Can you work these out from the model? Positions are in its coordinate system, mm. Face numbers are marked on the shaded views. Give positions to 0.01 mm unless a question says otherwise; leave off trailing zeros. Order: outer loops, then holes, each group sorted by start corner. A loop starts at its lowest first (then second) coordinate and runs counter-clockwise, first axis right, second up. Notation, with made-up numbers: (82.25, 23) -> (132.25, 23) arc R20 cw to (132.25, 29) -> close; hole circle Ø2 at (7.5, 86). An arc over 180 degrees is marked (long way). Answer as CSV lines item,"result".
```python
from build123d import *

# Parameters (mm, degrees)
EXTRUDE_1_DEPTH     = 20
SKETCH_2_R          = 1.5
CUT_EXTRUDE_1_DEPTH = 2.5


with BuildPart() as part:
    # 草图1 → 凸台-拉伸1 (new, symmetric)
    with BuildSketch(Plane.XY):
        Polygon((-4.5, 4.5), (4.5, 4.5), (4.5, 0), (13.5, 0), (13.5, 8), (-13.5, 8), (-13.5, 0), (-4.5, 0), align=None)
    extrude(amount=EXTRUDE_1_DEPTH, both=True)

    # 草图2 → 切除-拉伸1 (cut)
    with BuildSketch(Plane(origin=(0, 8, 0), x_dir=(1, 0, 0), z_dir=(0, 1, 0))):
        with Locations(Location((5, 12.5, 0), (0, 0, 180))):
            Circle(SKETCH_2_R)
        with Locations((-5, 12.5)):
            Circle(SKETCH_2_R)
        with Locations(Location((-5, -12.5, 0), (0, 0, 180))):
            Circle(SKETCH_2_R)
        with Locations((5, -12.5)):
            Circle(SKETCH_2_R)
    extrude(amount=-CUT_EXTRUDE_1_DEPTH, mode=Mode.SUBTRACT)


solid = part.part
```
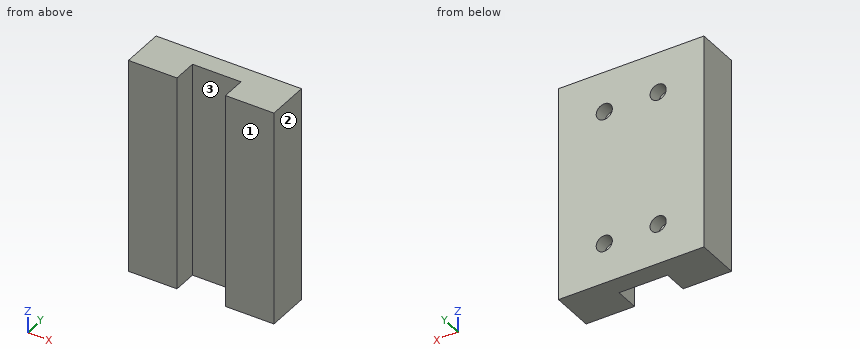
Item 1: Imagine slicing it at C-C, the plane y = 7.5. Please give me the cut outline in (x, z).
Numbers:
outline,"(-13.5, -20) -> (13.5, -20) -> (13.5, 20) -> (-13.5, 20) -> close; hole circle Ø3 at (-5, -12.5); hole circle Ø3 at (-5, 12.5); hole circle Ø3 at (5, -12.5); hole circle Ø3 at (5, 12.5)"
Item 2: We'd pull the mould along X, two halves only. Please class the marked faces 1, 2 and 3: released by +X, released by -X, zero draft, split by the parting line, or undercut.
Numbers:
face 1,"zero draft"
face 2,"released by +X"
face 3,"undercut"
Item 3: Imagine slicing it at A-A, the plane y = 2.5. Please give me the cut outline in (x, z).
Numbers:
outline,"(-13.5, -20) -> (-4.5, -20) -> (-4.5, 20) -> (-13.5, 20) -> close; (4.5, -20) -> (13.5, -20) -> (13.5, 20) -> (4.5, 20) -> close"
Item 4: Imagine slicing it at B-B, the plane x = -5. Please give me the cut outline in (y, z).
Numbers:
outline,"(0, -20) -> (8, -20) -> (8, -14) -> (5.5, -14) -> (5.5, -11) -> (8, -11) -> (8, 11) -> (5.5, 11) -> (5.5, 14) -> (8, 14) -> (8, 20) -> (0, 20) -> close"
Item 5: Imagine slicing it at D-D, the plane z = 4. Please give me the cut outline in (x, y).
Numbers:
outline,"(-13.5, 0) -> (-4.5, 0) -> (-4.5, 4.5) -> (4.5, 4.5) -> (4.5, 0) -> (13.5, 0) -> (13.5, 8) -> (-13.5, 8) -> close"
Item 6: For pin 1 (3.5 mm diameter, centred on x = -5.5, z = 12, fed in from +Y); pin 2 (0.9 mm diameter, centred on x = 5, z = -13, fed in from +Y); pin 3 (4.5 mm diameter, centred on x = 1, z = 3.5, fed in from -Y), each with a flat end and sliding along its axis, tell me the tip position at first contact or that it passes through.
Numbers:
pin 1,"stops at y = 8"
pin 2,"stops at y = 5.5"
pin 3,"stops at y = 4.5"
Item 7: Please list where these lines run through material, in increasing order: line 1 along Z through (x, y) = (5, 6.35); line 2 along X through (y, z) = (4, 6); line 3 along Y through (x, z) = (2, 13).
Numbers:
line 1,"z = -20 to -14, -11 to 11, 14 to 20"
line 2,"x = -13.5 to -4.5, 4.5 to 13.5"
line 3,"y = 4.5 to 8"
